CAD build for the part. Positions are in the model's coordinates, mm. Face numbers are marked on the shaded views. A direction names the side the tool comes from. Round coordinates to 2 decimals unless told otherwise and drop trailing zeros. Write each loop counter-clockwise with the first axis right and the second up, starting at its lowest first coordinate (ties: lowest second). Pieces come first, ordered by that corner, then holes. Notation, with made-up numbers: (0, 8) - (46, 8) arc R22 ccw to (46, 40) - close; hole circle Ø10 at (84, 71.25). An arc over 180 degrees is marked (long way). Answer in a Markdown table with one row per item.
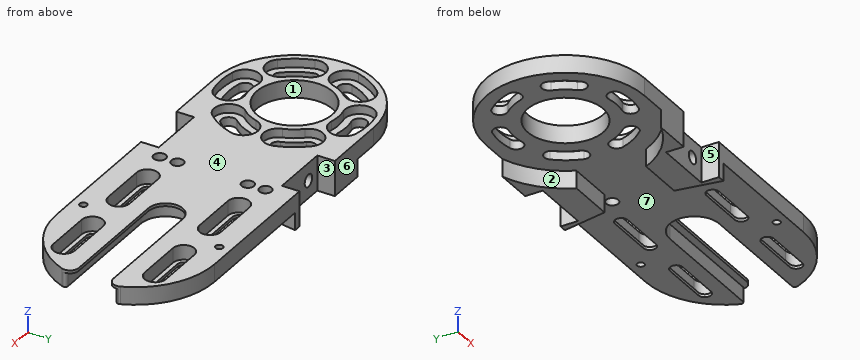
```python
from build123d import *

# Parameters (mm, degrees)
BOSS_EXTRUDE1_DEPTH            = 6
SKETCH2_R                      = 12.875
CUT_EXTRUDE1_DEPTH             = 78.129760793
CUT_EXTRUDE2_DEPTH             = 3
CUT_EXTRUDE3_DEPTH             = 78.129760793
CIRPATTERN1_COUNT              = 6
CUT_EXTRUDE4_DEPTH             = 5
FILLET1_R                      = 1
CUT_EXTRUDE5_DEPTH             = 78.129760793
FILLET2_R                      = 3
CUT_EXTRUDE6_DEPTH             = 5
CUT_EXTRUDE7_DEPTH             = 78.129760793
M3X0_5_TAPPED_HOLE1_D          = 2.5
M5X0_8_TAPPED_HOLE1_D          = 4.2
BOSS_EXTRUDE2_DEPTH            = 6
SKETCH15_W                     = 20
SKETCH15_H                     = 6
CUT_EXTRUDE8_DEPTH             = 78.826730626
M5X0_8_TAPPED_HOLE2_AT_2_COUNT = 2
M5X0_8_TAPPED_HOLE2_AT_2_PITCH = 10


with BuildPart() as part:
    # Sketch1 → Boss-Extrude1 (new body)
    with BuildSketch(Plane.XY):
        with BuildLine():
            Line((45, -27), (-45, -27))
            ThreePointArc((-45, -27), (-72, 0), (-45, 27))
            Line((-45, 27), (45, 27))
            ThreePointArc((45, 27), (72, 0), (45, -27))
        make_face()
    extrude(amount=BOSS_EXTRUDE1_DEPTH)

    # Sketch2 → Cut-Extrude1 (cut, through all)
    with BuildSketch(Plane.XY.offset(6)):
        with Locations((-45, 0)):
            Circle(SKETCH2_R)
    extrude(amount=-CUT_EXTRUDE1_DEPTH, mode=Mode.SUBTRACT)

    # Sketch3 → Cut-Extrude2 (cut)
    with BuildSketch(Plane.XY.offset(6)):
        with BuildLine():
            ThreePointArc((-39.507041214, 24.389083701), (-45, 25), (-50.492958786, 24.389083701))
            ThreePointArc((-50.492958786, 24.389083701), (-54.272183769, 18.412675204), (-48.295775272, 14.633450221))
            ThreePointArc((-48.295775272, 14.633450221), (-45, 15), (-41.704224728, 14.633450221))
            ThreePointArc((-41.704224728, 14.633450221), (-35.727816231, 18.412675204), (-39.507041214, 24.389083701))
        make_face()
    cut_extrude2 = extrude(amount=-CUT_EXTRUDE2_DEPTH, mode=Mode.SUBTRACT)

    # Sketch4 → Cut-Extrude3 (cut, through all)
    with BuildSketch(Plane.XY.offset(6)):
        with BuildLine():
            ThreePointArc((-40.056337093, 21.950175331), (-45, 22.5), (-49.943662907, 21.950175331))
            ThreePointArc((-49.943662907, 21.950175331), (-51.833275399, 18.961971082), (-48.84507115, 17.072358591))
            ThreePointArc((-48.84507115, 17.072358591), (-45, 17.5), (-41.15492885, 17.072358591))
            ThreePointArc((-41.15492885, 17.072358591), (-38.166724601, 18.961971082), (-40.056337093, 21.950175331))
        make_face()
    cut_extrude3 = extrude(amount=-CUT_EXTRUDE3_DEPTH, mode=Mode.SUBTRACT)

    # CirPattern1: Cut-Extrude2, Cut-Extrude3 ×6 about axis
    cirpattern1_axis = Axis((-45, 0, 0), (0, 0, 1))
    add([cut_extrude2.rotate(cirpattern1_axis, i * 360 / CIRPATTERN1_COUNT) for i in range(1, CIRPATTERN1_COUNT)], mode=Mode.SUBTRACT)
    add([cut_extrude3.rotate(cirpattern1_axis, i * 360 / CIRPATTERN1_COUNT) for i in range(1, CIRPATTERN1_COUNT)], mode=Mode.SUBTRACT)

    # Sketch5 → Cut-Extrude4 (cut)
    with BuildSketch(Plane(origin=(0, 0, 0), x_dir=(-1, 0, 0), z_dir=(0, 0, -1))):
        with BuildLine():
            Line((-72, 8.375), (-28, 8.375))
            ThreePointArc((-28, 8.375), (-19.625, 0), (-28, -8.375))
            Line((-28, -8.375), (-72, -8.375))
            ThreePointArc((-72, -8.375), (-80.375, 0), (-72, 8.375))
        make_face()
    extrude(amount=-CUT_EXTRUDE4_DEPTH, mode=Mode.SUBTRACT)

    # Fillet1
    fillet1_edges = [part.edges().sort_by_distance(p)[0] for p in [
        (70.668256174, 8.375, 2.5),
        (70.668256174, -8.375, 2.5),
    ]]
    fillet(fillet1_edges, radius=FILLET1_R)

    # Sketch6 → Cut-Extrude5 (cut, through all)
    with BuildSketch(Plane(origin=(0, 0, 0), x_dir=(-1, 0, 0), z_dir=(0, 0, -1))):
        with BuildLine():
            Line((-72, 5.875), (-28, 5.875))
            ThreePointArc((-28, 5.875), (-22.125, 0), (-28, -5.875))
            Line((-28, -5.875), (-72, -5.875))
            ThreePointArc((-72, -5.875), (-77.875, 0), (-72, 5.875))
        make_face()
    extrude(amount=-CUT_EXTRUDE5_DEPTH, mode=Mode.SUBTRACT)

    # Fillet2
    fillet2_edges = [part.edges().sort_by_distance(p)[0] for p in [
        (71.353071453, -5.875, 5.5),
        (71.353071453, 5.875, 5.5),
    ]]
    fillet(fillet2_edges, radius=FILLET2_R)

    # Sketch7 → Cut-Extrude6 (cut)
    with BuildSketch(Plane.XY.offset(6)):
        with BuildLine():
            Line((28.506349186, 11.906349186), (12.443650814, 11.906349186))
            ThreePointArc((12.443650814, 11.906349186), (8.793650814, 15.556349186), (12.443650814, 19.206349186))
            Line((12.443650814, 19.206349186), (28.506349186, 19.206349186))
            ThreePointArc((28.506349186, 19.206349186), (32.156349186, 15.556349186), (28.506349186, 11.906349186))
        make_face()
        with BuildLine():
            Line((59.619047558, 11.906349186), (43.556349186, 11.906349186))
            ThreePointArc((43.556349186, 11.906349186), (39.906349186, 15.556349186), (43.556349186, 19.206349186))
            Line((43.556349186, 19.206349186), (59.619047558, 19.206349186))
            ThreePointArc((59.619047558, 19.206349186), (63.269047558, 15.556349186), (59.619047558, 11.906349186))
        make_face()
    cut_extrude6 = extrude(amount=-CUT_EXTRUDE6_DEPTH, mode=Mode.SUBTRACT)

    # Sketch8 → Cut-Extrude7 (cut, through all)
    with BuildSketch(Plane.XY.offset(6)):
        with BuildLine():
            Line((12.443650814, 17.706349186), (28.506349186, 17.706349186))
            ThreePointArc((28.506349186, 17.706349186), (30.656349186, 15.556349186), (28.506349186, 13.406349186))
            Line((28.506349186, 13.406349186), (12.443650814, 13.406349186))
            ThreePointArc((12.443650814, 13.406349186), (10.293650814, 15.556349186), (12.443650814, 17.706349186))
        make_face()
        with BuildLine():
            Line((43.556349186, 17.706349186), (59.619047558, 17.706349186))
            ThreePointArc((59.619047558, 17.706349186), (61.769047558, 15.556349186), (59.619047558, 13.406349186))
            Line((59.619047558, 13.406349186), (43.556349186, 13.406349186))
            ThreePointArc((43.556349186, 13.406349186), (41.406349186, 15.556349186), (43.556349186, 17.706349186))
        make_face()
    cut_extrude7 = extrude(amount=-CUT_EXTRUDE7_DEPTH, mode=Mode.SUBTRACT)

    # M3x0.5 Tapped Hole1 (through all)
    with Locations(Plane.XY.offset(6)):
        with Locations((36.031349186, 23.15)):
            m3x0_5_tapped_hole1 = Hole(M3X0_5_TAPPED_HOLE1_D / 2)

    # M5x0.8 Tapped Hole1 (through all)
    with Locations(Plane.XY.offset(6)):
        with Locations((1.349738949, 12), (1.349738949, 18)):
            m5x0_8_tapped_hole1 = Hole(M5X0_8_TAPPED_HOLE1_D / 2)

    # Sketch14 → Boss-Extrude2 (add)
    with BuildSketch(Plane(origin=(0, 0, 0), x_dir=(-1, 0, 0), z_dir=(0, 0, -1))):
        with BuildLine():
            Line((0.5, 27), (3.166945583, 11.875))
            Line((3.166945583, 11.875), (19.091808728, 11.875))
            ThreePointArc((19.091808728, 11.875), (25.921018598, 21.171737498), (35.875856205, 27))
            Line((35.875856205, 27), (0.5, 27))
        make_face()
    boss_extrude2 = extrude(amount=BOSS_EXTRUDE2_DEPTH)

    # Sketch15 → Cut-Extrude8 (cut, through all)
    with BuildSketch(Plane.XY.offset(6)):
        with Locations((-13, 24)):
            Rectangle(SKETCH15_W, SKETCH15_H)
    cut_extrude8 = extrude(amount=-CUT_EXTRUDE8_DEPTH, mode=Mode.SUBTRACT)

    # Sketch17 → M5x0.8 Tapped Hole2 (revolve, cut)
    with BuildSketch(Plane(origin=(-18, 21, 0), x_dir=(0, 0, 1), z_dir=(1, 0, 0))):
        Polygon((0, 0), (0, 6.2618073), (2.1, 5), (2.1, 0), align=None)
    m5x0_8_tapped_hole2 = revolve(axis=Axis((-18, 27.35, 0), (0, -1, 0)), mode=Mode.SUBTRACT)

    # M5x0.8 Tapped Hole2 at 2: M5x0.8 Tapped Hole2 ×2
    with Locations(*[(i * M5X0_8_TAPPED_HOLE2_AT_2_PITCH, 0, 0) for i in range(1, M5X0_8_TAPPED_HOLE2_AT_2_COUNT)]):
        add(m5x0_8_tapped_hole2, mode=Mode.SUBTRACT)

    # Mirror1: Cut-Extrude6, Cut-Extrude7, M3x0.5 Tapped Hole1, M5x0.8 Tapped Hole1, Boss-Extrude2, Cut-Extrude8, M5x0.8 Tapped Hole2 across plane
    add(cut_extrude6.mirror(Plane.ZX), mode=Mode.SUBTRACT)
    add(cut_extrude7.mirror(Plane.ZX), mode=Mode.SUBTRACT)
    add(m3x0_5_tapped_hole1.mirror(Plane.ZX), mode=Mode.SUBTRACT)
    add(m5x0_8_tapped_hole1.mirror(Plane.ZX), mode=Mode.SUBTRACT)
    add(boss_extrude2.mirror(Plane.ZX))
    add(cut_extrude8.mirror(Plane.ZX), mode=Mode.SUBTRACT)
    add(m5x0_8_tapped_hole2.mirror(Plane.ZX), mode=Mode.SUBTRACT)

    # Mirror1 copy 1 sketch → Mirror1 copy 1 (revolve, cut)
    with BuildSketch(Plane(origin=(-8, -21, 0), x_dir=(0, 0, 1), z_dir=(1, 0, 0))):
        Polygon((0, 0), (0, -6.2618073), (2.1, -5), (2.1, 0), align=None)
    revolve(axis=Axis((-8, -27.35, 0), (0, -1, 0)), mode=Mode.SUBTRACT)


solid = part.part
```
Q1. 3-axis set-ups, long thin cutter, end or side, ignore diameter. For the marked faces 5, 6 and 7: which of +Z, -Z, +X, -X, +Y, -Y reach the whole face in a straight line?
Computed:
| item | result |
|---|---|
| face 5 | +Z, -Z, -Y |
| face 6 | +Z, -Z, +X, -X, +Y |
| face 7 | -Z |
Q2. Saw through at B-B on z = -3.5. List the corners of the cut face in (x, y) (3 decimals).
Computed:
| item | result |
|---|---|
| outline | (-35.876, -27) - (-23, -27) - (-23, -21) - (-3, -21) - (-3, -27) - (-0.5, -27) - (-3.167, -11.875) - (-19.092, -11.875) arc R28.5 cw to start; (-35.876, 27) arc R28.5 cw to (-19.092, 11.875) - (-3.167, 11.875) - (-0.5, 27) - (-3, 27) - (-3, 21) - (-23, 21) - (-23, 27) - close |
Q3. Pull direction X, two halves, no side cores. Call the marked faces 1, 2, 3 and 4: released by +X, released by -X, zero draft, split by the parting line, or undercut.
Computed:
| item | result |
|---|---|
| face 1 | undercut |
| face 2 | released by -X |
| face 3 | undercut |
| face 4 | zero draft |
Q4. Drill centre lines: line 1 (Y direction, x = -4, z = -4.75) (3 decimals); line 2 (Y direction, x = 57, z = 4.5) (3 decimals); line 3 (Y direction, x = -24.5, z = 5). Where is each one in solid material? Low to high.
Computed:
| item | result |
|---|---|
| line 1 | y = -21 to -11.875, 11.875 to 21 |
| line 2 | y = -24.187 to -19.206, -11.906 to -8.375, 8.375 to 11.906, 19.206 to 24.187 |
| line 3 | y = -27 to -14.31, -1.15 to 1.15, 14.31 to 27 |
Q5. Flat gauge pins, fed straight in: pin 1 (6 mm diameter, centred on y = -5, z = -1, fed in from -X); pin 2 (6 mm diameter, centred on x = 11.5, y = 8, fed in from -Z); pin 3 (7 mm diameter, centred on x = -31, y = 13.5, fed in from +Z). Where does each tip first touch, or does it go through?
Computed:
| item | result |
|---|---|
| pin 1 | stops at x = -71.91 |
| pin 2 | stops at z = 0 |
| pin 3 | stops at z = 3 |
Q6. Saw through at A-A on x = 17.5. List the corners of the cut face in (y, z), then the cut area to 3 significant figures.
Computed:
| item | result |
|---|---|
| outline | (-27, 0) - (-17.71, 0) - (-17.71, 1) - (-19.21, 1) - (-19.21, 6) - (-27, 6) - close; (-13.41, 0) - (13.41, 0) - (13.41, 1) - (11.91, 1) - (11.91, 6) - (-11.91, 6) - (-11.91, 1) - (-13.41, 1) - close; (17.71, 0) - (27, 0) - (27, 6) - (19.21, 6) - (19.21, 1) - (17.71, 1) - close |
| area | 242 mm2 |
